Autodesk Inventor part; units mm, degrees
ref_plane "YZ Plane" through (0, 0, 0) normal (1, 0, 0) x (0, 1, 0)
ref_plane "XZ Plane" through (0, 0, 0) normal (0, 1, 0) x (-1, 0, 0)
ref_plane "XY Plane" through (0, 0, 0) normal (0, 0, 1) x (1, 0, 0)
sketch "Boceto1" plane through (0, 0, 0) normal (0, 0, 1) x (1, 0, 0)
  circle A0 centre (0, -3.2) radius 3.2
  circle A1 centre (0, -3.2) radius 6.5
  circle A2 centre (0, -3.2) radius 9.5
  circle A3 centre (0, -3.2) radius 6.6
  line L0 (5.5183, 0.15) -> (15.5, 0.15)
  line L1 (15.5, 0.15) -> (15.5, -2.55)
  line L2 (15.5, -2.55) -> (5.5183, -2.55)
  line L3 (5.5183, -2.55) -> (5.5183, 0.15)
  line L4 (5.5183, -3.85) -> (15.5, -3.85)
  line L5 (15.5, -3.85) -> (15.5, -6.55)
  line L6 (15.5, -6.55) -> (5.5183, -6.55)
  line L7 (5.5183, -6.55) -> (5.5183, -3.85)
  line L8 (0, -3.2) -> (15.5144, -3.2)
  line L9 (9.5, -3.2) -> (9.5, 8.1404)
  arc A4 (9.2965, -1.2441) -> (-9.2965, -1.2441) centre (0, -3.2) ccw
  point P0 (0, 0)
  point P1 (8.8897, 0.15)
  point P2 (8.8897, -6.55)
  point P3 (6.4674, -3.85)
  point P4 (5.5702, -6.55)
  point P5 (5.6866, -6.55)
  point P6 (6.5679, -2.55)
  point P7 (6.5679, -3.85)
  dimension "d0" = 0.1
  dimension "d1" = 6
  dimension "d2" = 1.3
  dimension "d3" = 2.7
extrude "Extrusión1" add sketch "Boceto1" against normal blind 8 contours A3 L0 A2 L2 | L4 A2 L6 A3 | A3 L6 A2 L0 | A2 L0 L9 L2 | L4 L5 L6 A2 | L9 L0 L1 L2
sketch "Boceto2" plane through (8.8897, -6.55, 0) normal (0, -1, 0) x (1, 0, 0)
  line L0 (0, 0) -> (6.6103, 0)
  line L1 (0, 0) -> (0, -8)
  line L2 (6.6103, -8) -> (0, -8)
  line L3 (6.6103, 0) -> (6.6103, -8)
  line L4 (0, 0) -> (0, -8)
  line L5 (6.6103, 0) -> (6.6103, -8)
  line L6 (0, 0) -> (6.6103, -8)
  line L7 (1.3051, -2.8453) -> (3.3051, -1.6906)
  line L8 (3.3051, -1.6906) -> (5.3051, -2.8453)
  line L9 (5.3051, -2.8453) -> (5.3051, -5.1547)
  line L10 (5.3051, -5.1547) -> (3.3051, -6.3094)
  line L11 (3.3051, -6.3094) -> (1.3051, -5.1547)
  line L12 (1.3051, -5.1547) -> (1.3051, -2.8453)
  point P0 (-8.8897, 0)
  point P1 (3.3051, -4)
  dimension "d6" = 4
extrude "Extrusión2" cut sketch "Boceto2" against normal blind 1.35 contours L7 L8 L9 L10 L6 | L6 L10 L11 L12 L7
sketch "Boceto3" plane through (8.8897, -5.2, 0) normal (0, -1, 0) x (1, 0, 0)
  line L0 (3.3051, -6.3094) -> (1.3051, -5.1547)
  line L1 (5.3051, -2.8453) -> (1.3051, -5.1547)
  circle A0 centre (3.3051, -4) radius 1.1
  point P0 (-8.8897, 0)
  dimension "d9" = 2.2
extrude "Extrusión3" cut sketch "Boceto3" against normal through all
fillet "Empalme1" radius 3.5 4 edges at (15.5, -1.2, -8) (15.5, -5.2, -8) (15.5, -5.2, 0) (15.5, -1.2, 0)
properties part number "Cierre"
Check sheet for the modelled part. Datum: model origin and axes. Units: mm. A direction names the side the tool comes from. Round coordinates to 2 decimals unless told otherwise and drop trailing zeros. Order: outer loops, then holes, each group sorted by start corner. A loop starts at its lowest first (then second) coordinate and runs counter-clockwise, first axis right, second up.
1) Mould release check, pull along X, two halves, no side actions. Record for faces 1 (the cylindrical face through (14.45, -1.22, -7)), 2 (the flat face through (10, -3.85, -4)), 3 (the cylindrical face through (11.38, -4.53, -3.26)), 4 (the flat face through (13.209, -5.884, -5.724)): +X half, -X half, draft (parallel to the pull), parting line (faces both ways), or undercut.
2) Section check A-A (y = -4.5). Record the boundary of the cut face in (x, z).
3) Section check B-B (z = -4). Record the boundary of the cut face in (x, y).
4) Section check C-C (x = 3.25). Record the boundary of the cut face in (y, z).
5) Go/stop test with flat-tipped pins: pin 1 Ø2.5 at (x, z) = (10, -5.5) entering from -Y; pin 2 Ø1.3 at (x, z) = (12.19, -4) entering from +Y; pin 3 Ø2 at (x, z) = (11, -3) entering from -Y; pin 4 Ø3 at (y, z) = (-7.5, -4) entering from -X. Record where each tip stops, or that it passes through.
6) Scan lines: line 1 (Y direction, x = 11.75, z = -1.75); line 2 (X direction, y = -4.05, z = -4); line 3 (Y direction, x = 0, z = -4.5). Record each from-to range of solid material in increasing order.
7) Tool access check on faces 5 (the cylindrical face through (14.5, -1.22, -1.05)), 6 (the flat face through (11, 0.15, -5)), 7 (the flat face through (10, -2.55, -4)), 8 (the flat face through (10, -6.55, -4)), 9 (the flat face through (14.195, -6, -4)). Record the directions out of +Z, -Z, +X, -X, +Y, -Y that give a thin tool (end or side, any length) a straight path to the whole face; none if there is none.
8) Section check D-D (y = 2.75). Record the boundary of the cut face in (x, z).
Result:
1. face 1: +X half
1. face 2: draft
1. face 3: undercut
1. face 4: undercut
2. outline: (-9.41, -8) - (-6.47, -8) - (-6.47, 0) - (-9.41, 0) - close; (6.47, -8) - (12, -8) arc R3.5 ccw to (15.5, -4.5) - (15.5, -3.5) arc R3.5 ccw to (12, 0) - (6.47, 0) - close; hole circle Ø2.2 at (12.19, -4)
3. outline: (6.57, -3.85) arc R6.6 cw (long way) to (6.57, -2.55) - (11.09, -2.55) - (11.09, 0.15) - (8.89, 0.15) arc R9.5 ccw (long way) to (8.89, -6.55) - (10.19, -6.55) - (10.19, -5.2) - (11.09, -5.2) - (11.09, -3.85) - close; (13.29, -5.2) - (14.19, -5.2) - (14.19, -6.55) - (15.5, -6.55) - (15.5, -3.85) - (13.29, -3.85) - close; (13.29, -2.55) - (15.5, -2.55) - (15.5, 0.15) - (13.29, 0.15) - close
4. outline: (-12.13, -8) - (-8.94, -8) - (-8.94, 0) - (-12.13, 0) - close; (2.54, -8) - (5.73, -8) - (5.73, 0) - (2.54, 0) - close
5. pin 1: stops at y = -6.9
5. pin 2: passes through
5. pin 3: stops at y = -6.55
5. pin 4: stops at x = -9.08
6. line 1: y = -6.55 to -3.85, -2.55 to 0.15
6. line 2: x = -9.46 to -6.55, 6.55 to 11.09, 13.29 to 15.5
6. line 3: y = -12.7 to -9.8, 3.4 to 6.3
7. face 5: +Z, +X, +Y, -Y
7. face 6: +Z, -Z, +X, +Y
7. face 7: +Z, -Z, +X
7. face 8: +Z, -Z, +X, -Y
7. face 9: -Y
8. outline: (-7.41, -8) - (-2.86, -8) - (-2.86, 0) - (-7.41, 0) - close; (2.86, -8) - (7.41, -8) - (7.41, 0) - (2.86, 0) - close
